```python
from build123d import *

# Parameters (mm, degrees)
BOSS_EXTRUDE1_DEPTH     = 6
SKETCH2_W               = 100
SKETCH2_H               = 5.4
CUT_EXTRUDE_THIN1_DEPTH = 5
SKETCH3_OUTSIDE_W       = 132.574
SKETCH3_OUTSIDE_H       = 148.044
CUT_EXTRUDE1_DEPTH      = 6
INTERSECT1_START        = -50
INTERSECT1_DEPTH        = 50


# Read off the part's stored shape, not the designer's step: Intersect1
with BuildPart() as part:
    # Sketch1 → Boss-Extrude1 (new body)
    with BuildSketch(Plane(origin=(0, 0, 0), x_dir=(1, 0, 0), z_dir=(0, 1, 0))):
        Polygon((0, 57.735026919), (-50, 28.867513459), (-50, -28.867513459), (0, -57.735026919), (50, -28.867513459), (50, 28.867513459), align=None)
    extrude(amount=BOSS_EXTRUDE1_DEPTH)

    # Sketch2 → Cut-Extrude-Thin1 (cut)
    with BuildSketch(Plane.XZ):
        Polygon((-27.33826859, 41.951270189), (-3.33826859, 0.382050808), (1.33826859, 3.082050808), (-22.66173141, 44.651270189), align=None)
        Rectangle(SKETCH2_W, SKETCH2_H)
        Polygon((22.66173141, 44.651270189), (-1.33826859, 3.082050808), (3.33826859, 0.382050808), (27.33826859, 41.951270189), align=None)
    extrude(amount=-CUT_EXTRUDE_THIN1_DEPTH, mode=Mode.SUBTRACT)

    # Sketch3 outside → Cut-Extrude1 (cut)
    with BuildSketch(Plane.XZ):
        Rectangle(SKETCH3_OUTSIDE_W, SKETCH3_OUTSIDE_H)
        Polygon((-50, 28.867513459), (0, 57.735026919), (50, 28.867513459), (50, -4.7), (-50, -4.7), align=None, mode=Mode.SUBTRACT)
    extrude(amount=-CUT_EXTRUDE1_DEPTH, mode=Mode.SUBTRACT)

    # Intersect1 outline → Intersect1 (cut)
    with BuildSketch(Plane.YZ.offset(INTERSECT1_START)):
        Polygon((0, -2.7), (0, -4.7), (6, -4.7), (6, 59), (0, 59), (0, 2.7), (5, 2.7), (5, -2.7), align=None)
    extrude(amount=INTERSECT1_DEPTH, mode=Mode.SUBTRACT)


solid = part.part
```
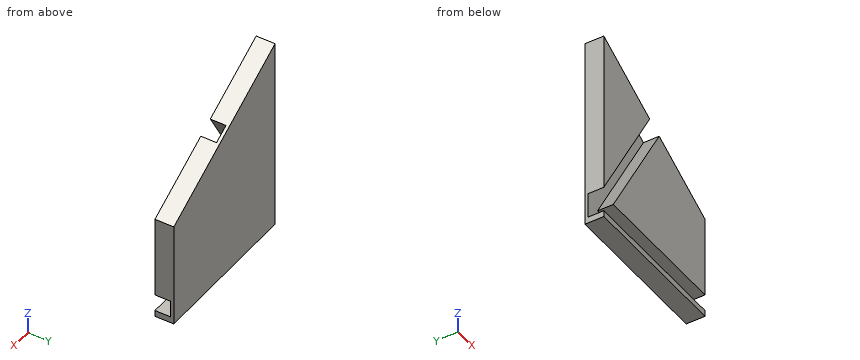
For this review, take the finished solid that the model builds, in its own axes (mm). Coordinates: 2 decimals unless noted, no trailing zeros. Order: outer loops, then holes, each group sorted by start corner. A loop starts at its lowest first (then second) coordinate and runs counter-clockwise, first axis right, second up. Notation, with made-up numbers: (-17.75, 26) - (34.25, 26) arc R20 cw to (34.25, 37) - close; hole circle Ø3 at (57.5, -37). An arc over 180 degrees is marked (long way). Answer as a JSON object with one key per item and string values. Group by question number.
1. For probe 1 along Z at (x, y) = (17.5, 2.3); probe 2 along Z at (x, y) = (6, 1.3); probe 3 along Y at (x, z) = (12, 18), list the stretches that pass through material, from the lowest coordinate up.
2. We need section D-D on z = 1. State the section outline as (x, y) points, then the cut area to 3 significant figures.
3. We need section B-B on z = 18.5. State the section outline as (x, y) points.
4. We need section C-C on x = 10. State the section outline as (y, z) points.
5. Clearance check with flat-ended pins moving along their axes: P1, Ø1.5, axis at x = 15, y = 2.5, coming from the +Z side; P2, Ø2, axis at x = 12.5, y = 3, coming from the +Z side. State where each tip first meets the part, or that it passes through.
6. We need section A-A on y = 3.25. State the section outline as (x, z) points, then the cut area to 3 significant figures.
Final values:
{
 "1": {"probe 1": "-4.7 to -2.7, 2.7 to 24.91, 35.71 to 47.63", "probe 2": "-4.7 to -2.7, 2.7 to 4.99, 15.79 to 54.27", "probe 3": "5 to 6"},
 "2": {"outline": "(0, 5) - (50, 5) - (50, 6) - (0, 6) - close", "area": "50.0 mm²"},
 "3": {"outline": "(0, 0) - (7.56, 0) - (7.56, 5) - (13.8, 5) - (13.8, 0) - (50, 0) - (50, 6) - (0, 6) - close"},
 "4": {"outline": "(0, -4.7) - (6, -4.7) - (6, 51.96) - (0, 51.96) - (0, 22.72) - (5, 22.72) - (5, 11.92) - (0, 11.92) - (0, 2.7) - (5, 2.7) - (5, -2.7) - (0, -2.7) - close"},
 "5": {"P1": "z = 49.51", "P2": "z = 51.1"},
 "6": {"outline": "(0, -4.7) - (50, -4.7) - (50, -2.7) - (0, -2.7) - close; (0, 5.4) - (22.66, 44.65) - (0, 57.74) - close; (4.68, 2.7) - (50, 2.7) - (50, 28.87) - (27.34, 41.95) - close", "area": "1,880 mm²"}
}
